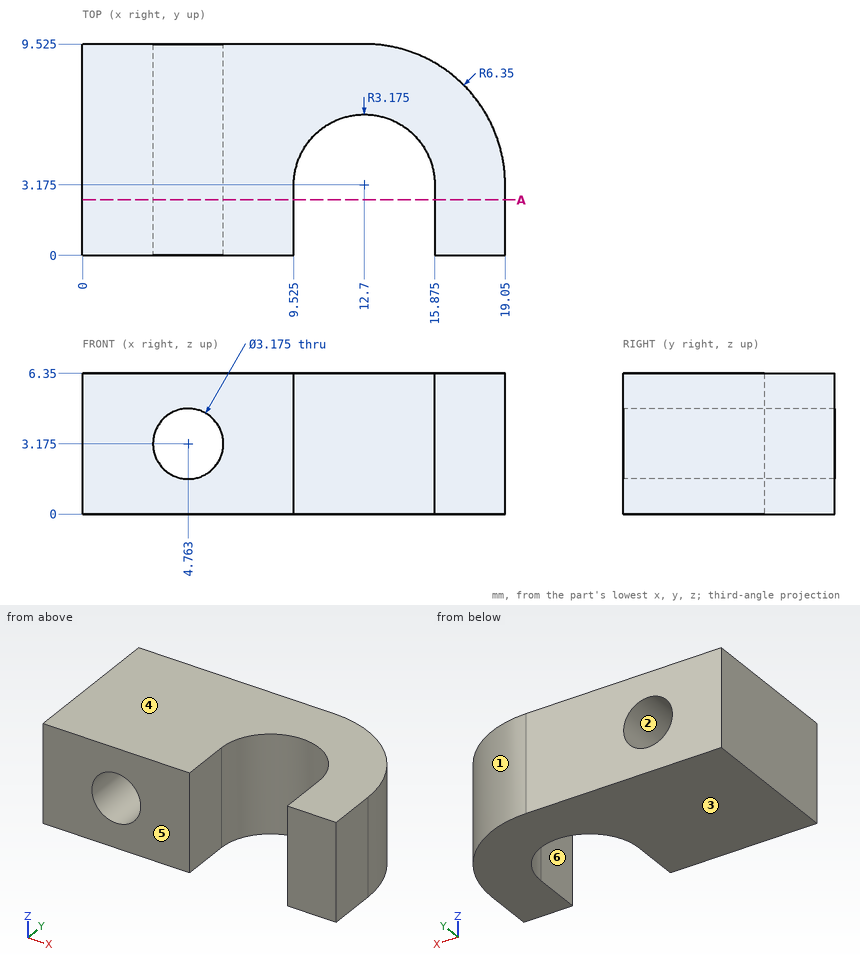
Source: three-view drawing plus pictorial views. Frame: mm from the lowest corner of the part. A direction names the side the tool comes from. Give positions to 0.01 mm unless a question says otherwise; leave off trailing zeros.
1) Line query: L1, parallel to X at y = 5.25, z = 4.5 (1 decimal); L2, parallel to X at y = 5.5, z = 3 (1 decimal); L3, parallel to X at y = 5.75, z = 1.5 (1 decimal). Output: solid intervals per line, ascending.
A:
L1: x = 0 to 3.9, 5.6 to 10.3, 15.1 to 18.7
L2: x = 0 to 3.2, 6.3 to 10.5, 14.9 to 18.6
L3: x = 0 to 10.8, 14.6 to 18.5
2) Mould query, pull axis Z, two halves, no side actions, for the marked faces 1, 2, 3 and 4. Classes: released by +Z, released by -Z, zero draft, split by the parting line, or undercut.
A:
face 1: zero draft
face 2: undercut
face 3: released by -Z
face 4: released by +Z
3) Reachability of the marked faces 5 and 6 from +Z, -Z, +X, -X, +Y, -Y: full face, straight path, thin tool, end or side. Return the list, or none.
A:
face 5: +Z, -Z, +X, -X, -Y
face 6: +Z, -Z, -Y
4) Section query A-A on y = 2.5. Count the separate pieces of the cut face and the enclosed holes in it.
A:
separate pieces: 2
enclosed holes: 1
5) Contact query for a flat-ended pin moving along its axis: pin 1 (2 mm diameter, centred on x = 13, y = 1.5, fed in from -Z). Output: stop coordinate, or through.
A:
pin 1: passes through
